from build123d import *

# Parameters (mm, degrees)
F0_R     = 19.05
F1_DEPTH = 38.1
F3_R     = 16.129
F4_DEPTH = 22.86
F5_R     = 17.145
F6_DEPTH = 53.34


with BuildPart() as f1:
    # F0 (on Top) → F1 (new body, symmetric)
    with BuildSketch(Plane.XY):
        Circle(F0_R)
    extrude(amount=F1_DEPTH, both=True)

    # F3 (on face) → F4 (cut)
    with BuildSketch(Plane(origin=(0, 0, -38.1), x_dir=(1, 0, 0), z_dir=(0, 0, -1))):
        Circle(F3_R)
    extrude(amount=-F4_DEPTH, mode=Mode.SUBTRACT)

    # F5 (on face) → F6 (cut)
    with BuildSketch(Plane.XY.offset(38.1)):
        Circle(F5_R)
    extrude(amount=-F6_DEPTH, mode=Mode.SUBTRACT)


solid = f1.part
Can you work these out from the model? Positions are in its coordinate system, mm. A direction names the side the tool comes from. Give positions to 0.01 mm unless a question says otherwise; leave off trailing zeros. Write each loop counter-clockwise with the first axis right and the second up, starting at its lowest first coordinate (ties: lowest second). Pieces come first, ordered by that corner, then holes. Notation, with made-up numbers: (17.5, 2.25) -> (45.5, 2.25) arc R6 cw to (45.5, 13.25) -> close; hole circle Ø11 at (82.25, 41.5). An arc over 180 degrees is marked (long way). Answer as a JSON object with one key per item and string values. Group by question number.
Item 1: For faces 1 (the face through (9.217, 14.457, 11.803)), 2 (the face through (15.4, -4.8, -26.8)), which set-ups out of +Z, -Z, +X, -X, +Y, -Y let a thin tool reach every point of the face, with its end or its side?
Item 2: Suppose I cut it at C-C (z = -28). Please give me the cut outline in (x, y).
Item 3: Suppose I cut it at A-A (y = 0). Please give me the cut outline in (x, z) (3 decimals).
Item 4: Please list where these lines run through material, in increasing order: line 1 (Y direction, x = 0, z = 6) (3 decimals); line 2 (Y direction, x = 0, z = -24); line 3 (X direction, y = -14, z = -28). Write a range as [from, to].
Item 5: I'm going to push flat-ended pins straight in: P1, Ø5, axis at x = 10.5, z = 28.5, coming from the -Y side; P2, Ø12, axis at y = -12.5, z = -28, coming from the -X side; P3, Ø1.5, axis at x = 12.5, y = 8, coming from the -Z side; P4, Ø6, axis at x = -1, y = 14, coming from the +Z side. Where does each tip first touch, or does it pass through?
Item 6: We'd pull the mould along X, two halves only. Please class faces 3 (the face through (13, -10, -15.24)), 4 (the face through (-16, 4, -38.1)), 5 (the face through (-15.12, -11.59, 0.53)): +X half, -X half, draft (parallel to the pull), parting line (faces both ways), or undercut.
Item 7: Suppose I cut it at D-D (z = 8.5). Please give me the cut outline in (x, y) (3 decimals), plus the area to 3 significant figures.
Findings:
{
 "1": {"face 1": "+Z", "face 2": "+Z, -Z"},
 "2": {"outline": "circle Ø38.1 at (0, 0); hole circle Ø32.26 at (0, 0)"},
 "3": {"outline": "(-19.05, -38.1) -> (-16.129, -38.1) -> (-16.129, -15.24) -> (-17.145, -15.24) -> (-17.145, 38.1) -> (-19.05, 38.1) -> close; (16.129, -38.1) -> (19.05, -38.1) -> (19.05, 38.1) -> (17.145, 38.1) -> (17.145, -15.24) -> (16.129, -15.24) -> close"},
 "4": {"line 1": "y = [-19.05, -17.145], [17.145, 19.05]", "line 2": "y = [-19.05, -16.13], [16.13, 19.05]", "line 3": "x = [-12.92, -8.01], [8.01, 12.92]"},
 "5": {"P1": "stops at y = -17.29", "P2": "stops at x = -17.91", "P3": "passes through", "P4": "stops at z = -15.24"},
 "6": {"face 3": "undercut", "face 4": "draft", "face 5": "parting line"},
 "7": {"outline": "circle Ø38.1 at (0, 0); hole circle Ø34.29 at (0, 0)", "area": "217 mm²"}
}
